Verification items for the finished model (mm, model axes). A direction names the side the tool comes from. Give positions to 0.01 mm unless a question says otherwise; leave off trailing zeros. Loops run counter-clockwise (first coordinate to the right, second up) from the corner with the lowest first, then second, coordinate; pieces in that order, holes last. Notation, with made-up numbers: M -15.5,2 L 38.5,2 A21 cw 38.5,12 Z; hole C 30,12.5 d1. An arc over 180 degrees is marked long. Use a Markdown table: item, result.
from build123d import *

# Parameters (mm, degrees)
F0_R     = 2.75
F0_R_2   = 14
F0_R_3   = 8
F1_DEPTH = 10
F2_DEPTH = 36
F3_SIZE  = 0.5


with BuildPart() as f1:
    # F0 (on Top) → F1 (new body)
    with BuildSketch(Plane.XY):
        with BuildLine():
            Line((20, -13.266499), (20, 13.266499))
            ThreePointArc((20, 13.266499), (0, 24), (-20, 13.266499))
            Line((-20, 13.266499), (-20, -13.266499))
            ThreePointArc((-20, -13.266499), (0, -24), (20, -13.266499))
        make_face()
        with Locations((-13.435029, -13.435029)):
            Circle(F0_R, mode=Mode.SUBTRACT)
        with Locations((0, -19)):
            Circle(F0_R, mode=Mode.SUBTRACT)
        with Locations((13.435029, -13.435029)):
            Circle(F0_R, mode=Mode.SUBTRACT)
        with Locations((-13.435029, 13.435029)):
            Circle(F0_R, mode=Mode.SUBTRACT)
        Circle(F0_R_2, mode=Mode.SUBTRACT)
        with Locations((0, 19)):
            Circle(F0_R, mode=Mode.SUBTRACT)
        with Locations((13.435029, 13.435029)):
            Circle(F0_R, mode=Mode.SUBTRACT)
        Circle(F0_R_2)
        Circle(F0_R_3, mode=Mode.SUBTRACT)
    extrude(amount=-F1_DEPTH)

    # F0 (on Top) → F2 (join)
    with BuildSketch(Plane.XY):
        Circle(F0_R_2)
        Circle(F0_R_3, mode=Mode.SUBTRACT)
    extrude(amount=-F2_DEPTH)

    # F3
    f3_edges = [f1.edges().sort_by_distance(p)[0] for p in [
        (-14, 0, -36),
    ]]
    chamfer(f3_edges, length=F3_SIZE)


solid = f1.part
(1) Material ranges on line 1 (Y direction, x = 12, z = -9.5); line 2 (Z direction, x = 4, y = -20); line 3 (Y direction, x = -1, z = -4), recorded low to high.
Results below:
| item | result |
|---|---|
| line 1 | -20.78 to -15.78, -11.09 to 11.09, 15.78 to 20.78 |
| line 2 | -10 to 0 |
| line 3 | -23.98 to -21.56, -16.44 to -7.94, 7.94 to 16.44, 21.56 to 23.98 |
(2) Set-up check for faces 1 (the flat face through (-9, 11, -10)), 2 (the cylindrical face through (-16.182, 13.556, -4.93)): record each of +Z, -Z, +X, -X, +Y, -Y from which the full face is reachable in a straight line by a thin tool's end or side.
Results below:
| item | result |
|---|---|
| face 1 | -Z |
| face 2 | +Z, -Z |
(3) Cross-section at A-A on x = 0. Record the cut outline in (y, z), then the cut area to 3 significant figures.
Results below:
| item | result |
|---|---|
| outline | M -24,-10 L -21.75,-10 L -21.75,0 L -24,0 Z; M -16.25,-10 L -14,-10 L -14,-35.5 L -13.5,-36 L -8,-36 L -8,0 L -16.25,0 Z; M 8,-36 L 13.5,-36 L 14,-35.5 L 14,-10 L 16.25,-10 L 16.25,0 L 8,0 Z; M 21.75,-10 L 24,-10 L 24,0 L 21.75,0 Z |
| area | 522 mm^2 |
(4) Cross-section at D-D on y = 20. Record the cut outline in (x, z), then the cut area to 3 significant figures.
Results below:
| item | result |
|---|---|
| outline | M -13.27,-10 L -2.56,-10 L -2.56,0 L -13.27,0 Z; M 2.56,-10 L 13.27,-10 L 13.27,0 L 2.56,0 Z |
| area | 214 mm^2 |
(5) Cross-section at C-C on z = -3. Record the cut outline in (x, y), then the cut area to 3 significant figures.
Results below:
| item | result |
|---|---|
| outline | M -20,-13.27 A24 ccw 20,-13.27 L 20,13.27 A24 ccw -20,13.27 Z; hole C -13.44,-13.44 d5.5; hole C -13.44,13.44 d5.5; hole C 0,0 d16; hole C 0,-19 d5.5; hole C 0,19 d5.5; hole C 13.44,-13.44 d5.5; hole C 13.44,13.44 d5.5 |
| area | 1,320 mm^2 |
(6) Gauge pin test, flat ends, axial feed: P1, Ø3, axis at x = 2, z = -9.5, coming from the +Y side; P2, Ø9.5, axis at x = 0, y = 0, coming from the +Z side; P3, Ø9, axis at x = 13.44, y = 13.44, coming from the -Z side; P4, Ø4, axis at y = 2, z = -29.5, coming from the +X side. Record the tip position at first contact, or that the pin passes through.
Results below:
| item | result |
|---|---|
| P1 | y = 23.99 |
| P2 | through |
| P3 | z = -10 |
| P4 | x = 14 |
(7) Draft check along Y on faces 3 (the cylindrical face through (-0.358, 21.727, -4.93)), 4 (the flat face through (9, 0, 0)), 5 (the cylindrical face through (12.932, -5.362, -22.572)). Enter one of: +Y half, -Y half, draft (parallel to the pull), parting line (faces both ways), or undercut.
Results below:
| item | result |
|---|---|
| face 3 | undercut |
| face 4 | draft |
| face 5 | parting line |
(8) Cross-section at B-B on y = 0. Record the cut outline in (x, z), then the cut area to 3 significant figures.
Results below:
| item | result |
|---|---|
| outline | M -20,-10 L -14,-10 L -14,-35.5 L -13.5,-36 L -8,-36 L -8,0 L -20,0 Z; M 8,-36 L 13.5,-36 L 14,-35.5 L 14,-10 L 20,-10 L 20,0 L 8,0 Z |
| area | 552 mm^2 |
